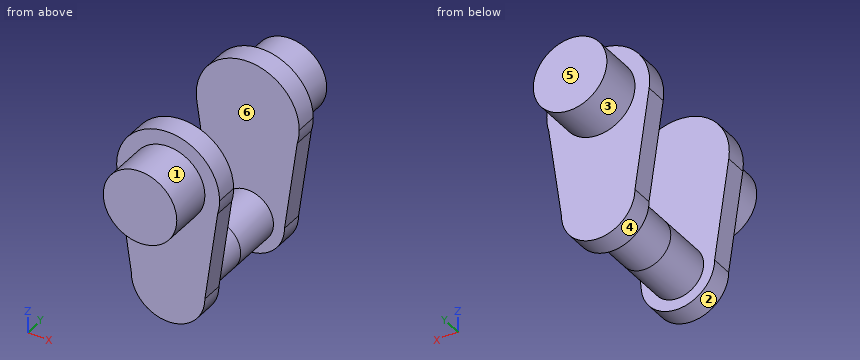
from build123d import *

# Parameters (mm, degrees)
F1_DEPTH = 38.1
F2_R     = 63.5
F3_DEPTH = 76.2
F4_R     = 44.45
F5_DEPTH = 88.9


with BuildPart() as f1:
    # F0 (on Front) → F1 (new body)
    with BuildSketch(Plane.XZ):
        with BuildLine():
            Line((88.9, 0), (85.51811, -24.287093))
            ThreePointArc((85.51811, -24.287093), (88.050468, -12.260711), (88.9, 0))
        make_face()
        with BuildLine():
            Line((63.5, -182.410464), (85.51811, -24.287093))
            Line((85.51811, -24.287093), (88.9, 0))
            ThreePointArc((88.9, 0), (-6.364448, 88.671888), (-87.988724, -12.696234))
            Line((-87.988724, -12.696234), (-63.5, -182.410464))
            ThreePointArc((-63.5, -182.410464), (0, -245.910464), (63.5, -182.410464))
        make_face()
    extrude(amount=F1_DEPTH)

    # F2 (on face) → F3 (join)
    with BuildSketch(Plane.XZ.offset(38.1)):
        Circle(F2_R)
    extrude(amount=F3_DEPTH)

    # F4 (on face) → F5 (join)
    with BuildSketch(Plane(origin=(0, 0, 0), x_dir=(-1, 0, 0), z_dir=(0, 1, 0))):
        with Locations((0, -182.410464)):
            Circle(F4_R)
    extrude(amount=F5_DEPTH)

    # F6: F1 across face


with BuildPart() as f1_1:
    add(f1.part)
    add(f1.part.mirror(Plane(origin=(0, 88.9, -182.410464), x_dir=(-1, 0, 0), z_dir=(0, 1, 0))))


solid = f1_1.part
Source: CAD feature listing. Evaluate the final solid. Frame: model axes, mm. Face numbers are marked on the shaded views. A direction names the side the tool comes from. Coordinates: 2 decimals unless noted, no trailing zeros. Loops run counter-clockwise (first coordinate to the right, second up) from the corner with the lowest first, then second, coordinate; pieces in that order, holes last. Notation, with made-up numbers: (54.5, 70) -> (83.5, 70) arc R24 ccw to (83.5, 80) -> close; hole circle Ø10 at (-28.5, -35.75). An arc over 180 degrees is marked (long way). Answer in a Markdown table with one row per item. Add a question column.
Q1. Section D-D on y = 207. Return the cut outline in (x, z).
Q2. Section A-A on z = -59. Return the cut outline in (x, y), and give its area (3 significant figures).
Q3. Section B-B on x = -72. Return the cut outline in (y, z), and give its area (3 significant figures).
Q4. Ray query, line 1 along Y through (x, z) = (-60.5, -164); line 2 along Y through (x, z) = (-35.5, 9); line 3 along X through (y, z) = (27, -185). Return the intervals inside material, ascending.
Q5. Reachability of the marked faces 1, 2 and 3 from +Z, -Z, +X, -X, +Y, -Y: full face, straight path, thin tool, end or side. Return the list, or none.
Q6. Section C-C on x = 0. Return the cut outline in (y, z), and give its area (3 significant figures).
Q7. Pull-direction query (Y, two-part tool) for the marked faces 4, 5 and 6; classes: pulls with the +Y half, pulls with the -Y half, needs draft (parallel to the pull), parting line crosses it, or undercut.
Q8. Contact query for flat-ended pins moving along their axis: pin 1 Ø6 at (x, z) = (-68.5, -173) entering from +Y; pin 2 Ø10 at (x, y) = (-56, 217) entering from -Z; pin 3 Ø10 at (x, y) = (-34, -41.5) entering from -Z; pin 4 Ø12 at (x, z) = (40.5, -153) entering from -Y. Output: stop coordinate, or through.
Computed values:
| question | item | result |
|---|---|---|
| 1 | outline | (-87.99, -12.7) -> (-63.5, -182.41) arc R63.5 ccw to (63.5, -182.41) -> (85.52, -24.29) arc R88.9 ccw to (88.9, 0) arc R88.9 ccw (long way) to start |
| 2 | outline | (-81.31, -38.1) -> (-23.48, -38.1) -> (-23.48, -114.3) -> (23.48, -114.3) -> (23.48, -38.1) -> (80.68, -38.1) -> (80.68, 0) -> (-81.31, 0) -> close; (-81.31, 177.8) -> (80.68, 177.8) -> (80.68, 215.9) -> (23.48, 215.9) -> (23.48, 292.1) -> (-23.48, 292.1) -> (-23.48, 215.9) -> (-81.31, 215.9) -> close |
| 2 | area | 19,500 mm^2 |
| 3 | outline | (-38.1, -123.5) -> (0, -123.5) -> (0, 52.15) -> (-38.1, 52.15) -> close; (177.8, -123.5) -> (215.9, -123.5) -> (215.9, 52.15) -> (177.8, 52.15) -> close |
| 3 | area | 13,400 mm^2 |
| 4 | line 1 | y = -38.1 to 0, 177.8 to 215.9 |
| 4 | line 2 | y = -114.3 to 0, 177.8 to 292.1 |
| 4 | line 3 | x = -44.37 to 44.37 |
| 5 | face 1 | -Y |
| 5 | face 2 | -Z, +Y, -Y |
| 5 | face 3 | +Y |
| 6 | outline | (-114.3, -63.5) -> (-38.1, -63.5) -> (-38.1, -245.91) -> (0, -245.91) -> (0, -226.86) -> (177.8, -226.86) -> (177.8, -245.91) -> (215.9, -245.91) -> (215.9, -63.5) -> (292.1, -63.5) -> (292.1, 63.5) -> (215.9, 63.5) -> (215.9, 88.9) -> (177.8, 88.9) -> (177.8, -137.96) -> (0, -137.96) -> (0, 88.9) -> (-38.1, 88.9) -> (-38.1, 63.5) -> (-114.3, 63.5) -> close |
| 6 | area | 60,700 mm^2 |
| 7 | face 4 | needs draft |
| 7 | face 5 | pulls with the +Y half |
| 7 | face 6 | undercut |
| 8 | pin 1 | passes through |
| 8 | pin 2 | stops at z = -220.08 |
| 8 | pin 3 | stops at z = -238.2 |
| 8 | pin 4 | stops at y = -38.1 |
